Geometry: final body of the model. Coordinates: model frame, mm. Face numbers are marked on the shaded views. A direction names the side the tool comes from. Round coordinates to 2 decimals unless told otherwise and drop trailing zeros. Write each loop counter-clockwise with the first axis right and the second up, starting at its lowest first coordinate (ties: lowest second). Pieces come first, ordered by that corner, then holes. Notation, with made-up numbers: M 56.25,69.5 L 111.25,69.5 A10 cw 111.25,88.5 Z; hole C 63.5,66.5 d8. An arc over 180 degrees is marked long. Use one line per item in the form item = value. Start each with the question number.
Item 1: Pull-direction query (X, two-part tool) for the marked faces 4, 5 and 6; classes: pulls with the +X half, pulls with the -X half, needs draft (parallel to the pull), parting line crosses it, or undercut.
Item 2: Reachability of the marked faces 1, 2 and 3 from +Z, -Z, +X, -X, +Y, -Y: full face, straight path, thin tool, end or side. Return the list, or none.
Item 3: Section query B-B (y = 0). Return loops of the section in (x, z).
Item 4: Ray query, probe 1 along Y at (x, z) = (1, 1.5); probe 2 along X at (y, z) = (17, 4); probe 3 along Y at (x, z) = (-6, 4.5). Return the intervals inside material, ascending.
Item 5: Section query C-C (z = 1.25). Return loops of the section in (x, y).
Item 6: Section query A-A (x = 0). Return loops of the section in (y, z).
Item 7: Section query D-D (x = -14). Return loops of the section in (y, z), and give its area (3 significant figures).
Item 8: Pin query (flat end, axial travel): pin 1 Ø1.5 at (x, z) = (15.5, 7.5) entering from +Y; pin 2 Ø2.5 at (y, z) = (17, 3) entering from -X; pin 3 Ø4 at (y, z) = (-2.5, 5.5) entering from +X; pin 4 Ø12 at (x, y) = (14, 0.5) entering from +Z. Return the tip coordinate at first contact, or that it passes through.
from build123d import *

# Parameters (mm, degrees)
RESSALTO_EXTRUS_O2_DEPTH = 6
CORTE_EXTRUS_O1_DEPTH    = 1
ESBO_O8_W                = 3
ESBO_O8_H                = 3
RESSALTO_EXTRUS_O4_DEPTH = 6
RESSALTO_EXTRUS_O5_DEPTH = 4


with BuildPart() as part:
    # Esboço4 → Ressalto-extrusão2 (new body)
    with BuildSketch(Plane.XY):
        with BuildLine():
            Line((10.25, 17.753520778), (8.3, 14.376021703))
            ThreePointArc((8.3, 14.376021703), (16.535747837, -1.45912421), (5.654249214, -15.607352941))
            ThreePointArc((5.654249214, -15.607352941), (1.575368798, -19.389491614), (-3.857534027, -18.195588235))
            ThreePointArc((-3.857534027, -18.195588235), (-17.949080324, 4.877552207), (5.882044961, 17.645439838))
            Line((5.882044961, 17.645439838), (6.482899016, 19.447931004))
            ThreePointArc((6.482899016, 19.447931004), (-8.409235035, -18.695848901), (10.25, 17.753520778))
        make_face()
    extrude(amount=RESSALTO_EXTRUS_O2_DEPTH)

    # Esboço7 → Corte-extrusão1 (cut)
    with BuildSketch(Plane.XY.offset(6)):
        with BuildLine():
            Line((-3.857534027, -18.195588235), (-4.251583202, -20.054277356))
            ThreePointArc((-4.251583202, -20.054277356), (19.140340931, -7.341481393), (10.25, 17.753520778))
            Line((10.25, 17.753520778), (8.3, 14.376021703))
            ThreePointArc((8.3, 14.376021703), (16.535747837, -1.45912421), (5.654249214, -15.607352941))
            ThreePointArc((5.654249214, -15.607352941), (1.575368798, -19.389491614), (-3.857534027, -18.195588235))
        make_face()
    extrude(amount=-CORTE_EXTRUS_O1_DEPTH, mode=Mode.SUBTRACT)

    # Esboço8 → Ressalto-extrusão4 (add)
    with BuildSketch(Plane(origin=(0, 0, 0), x_dir=(-1, 0, 0), z_dir=(0, 0, -1))):
        with BuildLine():
            ThreePointArc((9.976510425, -11.876705547), (4.856795522, -10.085239821), (3.065329796, -15.204954723))
            Line((3.065329796, -15.204954723), (5.002459987, -19.227447012))
            Line((5.002459987, -19.227447012), (11.913640616, -15.899197835))
            Line((11.913640616, -15.899197835), (9.976510425, -11.876705547))
        make_face()
        Polygon((5.820292417, -15.543109046), (4.5186412, -12.840202442), (7.221547804, -11.538551224), (8.523199021, -14.241457828), align=None, mode=Mode.SUBTRACT)
        with BuildLine():
            ThreePointArc((-3.835415892, 15.029187597), (0, 11.193771705), (3.835415892, 15.029187597))
            Line((3.835415892, 15.029187597), (3.835415892, 19.493817211))
            Line((3.835415892, 19.493817211), (-3.835415892, 19.493817211))
            Line((-3.835415892, 19.493817211), (-3.835415892, 15.029187597))
        make_face()
        with Locations((0, 15.029187597)):
            Rectangle(ESBO_O8_W, ESBO_O8_H, mode=Mode.SUBTRACT)
    extrude(amount=-RESSALTO_EXTRUS_O4_DEPTH)

    # Esboço9 → Ressalto-extrusão5 (add)
    with BuildSketch(Plane.XY.offset(6)):
        with BuildLine():
            Line((-4.0441889, -19.076019924), (-4.251583202, -20.054277356))
            ThreePointArc((-4.251583202, -20.054277356), (-19.782588529, 5.375796787), (6.482899016, 19.447931004))
            Line((6.482899016, 19.447931004), (6.16666004, 18.499251443))
            ThreePointArc((6.16666004, 18.499251443), (-18.81758421, 5.113562798), (-4.0441889, -19.076019924))
        make_face()
    extrude(amount=RESSALTO_EXTRUS_O5_DEPTH)


solid = part.part
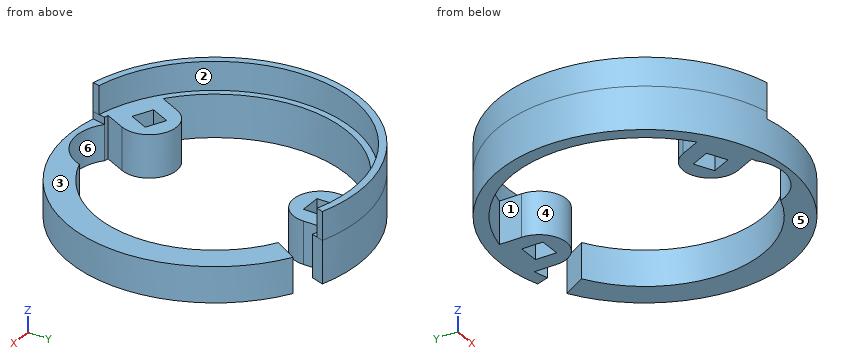
Working result:
q1.face_4 = undercut
q1.face_5 = needs draft
q1.face_6 = undercut
q2.face_1 = +Z, -Z
q2.face_2 = +Z
q2.face_3 = +Z, +X, -Y
q3.outline = M -20.5,0 L -18.6,0 L -18.6,6 L -19.5,6 L -19.5,10 L -20.5,10 Z; M 16.6,0 L 20.5,0 L 20.5,5 L 16.6,5 Z
q4.probe_1 = -20.48 to -19.52, 11.33 to 13.53, 16.53 to 20.48
q4.probe_2 = -11.46 to -7.55, -3.84 to 3.84, 9.81 to 11.46
q4.probe_3 = -19.6 to -15.46, -12.13 to -9.74, 17.61 to 19.6
q5.outline = M -11.35,-14.73 A18.6 cw -3.84,18.2 L -3.84,15.03 A3.84 ccw 3.84,15.03 L 3.84,18.2 A18.6 cw 5.88,17.65 L 6.48,19.45 A20.5 ccw long 10.25,17.75 L 8.3,14.38 A16.6 cw 5.65,-15.61 A6 cw -3.86,-18.2 A18.6 cw -4.44,-18.06 L -3.07,-15.2 A3.84 ccw -9.98,-11.88 Z; hole M -8.52,-14.24 L -5.82,-15.54 L -4.52,-12.84 L -7.22,-11.54 Z; hole M -1.5,13.53 L 1.5,13.53 L 1.5,16.53 L -1.5,16.53 Z
q6.outline = M -20.5,0 L -19.6,0 L -19.6,5 L -20.5,5 Z; M 11.19,0 L 13.53,0 L 13.53,6 L 11.19,6 Z; M 16.53,0 L 20.5,0 L 20.5,10 L 19.5,10 L 19.5,6 L 16.53,6 Z
q7.outline = M -14.97,0 L -12.25,0 L -12.25,6 L -13.57,6 L -13.57,10 L -14.97,10 Z; M 12.25,0 L 14.97,0 L 14.97,10 L 13.57,10 L 13.57,6 L 12.25,6 Z
q7.area = 44.0 mm²
q8.pin_1 = through
q8.pin_2 = -13.12
q8.pin_3 = 20.49
q8.pin_4 = 5
